```python
from build123d import *

# Parameters (mm, degrees)
SKETCH_8_W              = 3.5
SKETCH_8_H              = 303
SM_BASE_FLANGE_3_DEPTH  = 1.5
SM_EDGE_FLANGE_4_DEPTH  = 303
SM_EDGE_FLANGE_9_DEPTH  = 303
SM_EDGE_FLANGE_10_DEPTH = 303
FILLET_1_R              = 2


# Sheet-metal steps are written as plain solids
with BuildPart() as part:
    # Эскиз8 → Базовая кромка3 (new body)
    with BuildSketch(Plane.XY):
        with Locations((1.75, 151.5)):
            Rectangle(SKETCH_8_W, SKETCH_8_H)
    extrude(amount=-SM_BASE_FLANGE_3_DEPTH)

    # Ребро-кромка4 section (across the edge) → Ребро-кромка4 (add)
    with BuildSketch(Plane(origin=(32, 0, 0), x_dir=(-1, 0, 0), z_dir=(0, 1, 0))):
        with BuildLine():
            Line((-1.5, 28.5), (-1.5, 35))
            Line((-1.5, 35), (0, 35))
            Line((0, 35), (0, 28.5))
            ThreePointArc((0, 28.5), (8.347456736, 8.347456736), (28.5, 0))
            Line((28.5, 0), (28.5, -1.5))
            ThreePointArc((28.5, -1.5), (7.286796564, 7.286796564), (-1.5, 28.5))
        make_face()
    extrude(amount=SM_EDGE_FLANGE_4_DEPTH)

    # Ребро-кромка9 section (across the edge) → Ребро-кромка9 (add)
    with BuildSketch(Plane(origin=(-2, 303, 0), x_dir=(1, 0, 0), z_dir=(0, -1, 0))):
        with BuildLine():
            Line((-1.5, 2), (-1.5, 16.5))
            Line((-1.5, 16.5), (0, 16.5))
            Line((0, 16.5), (0, 2))
            ThreePointArc((0, 2), (0.585786438, 0.585786438), (2, 0))
            Line((2, 0), (2, -1.5))
            ThreePointArc((2, -1.5), (-0.474873734, -0.474873734), (-1.5, 2))
        make_face()
    extrude(amount=SM_EDGE_FLANGE_9_DEPTH)

    # Ребро-кромка10 section (across the edge) → Ребро-кромка10 (add)
    with BuildSketch(Plane(origin=(32, 0, 37), x_dir=(0, 0, -1), z_dir=(0, 1, 0))):
        with BuildLine():
            Line((-1.5, 2), (-1.5, 16.5))
            Line((-1.5, 16.5), (0, 16.5))
            Line((0, 16.5), (0, 2))
            ThreePointArc((0, 2), (0.585786438, 0.585786438), (2, 0))
            Line((2, 0), (2, -1.5))
            ThreePointArc((2, -1.5), (-0.474873734, -0.474873734), (-1.5, 2))
        make_face()
    extrude(amount=SM_EDGE_FLANGE_10_DEPTH)

    # Скругление1
    fillet_1_edges = [part.edges().sort_by_distance(p)[0] for p in [
        (-2.75, 303, 16.5),
        (-2.75, 0, 16.5),
        (15.5, 0, 37.75),
        (15.5, 303, 37.75),
    ]]
    fillet(fillet_1_edges, radius=FILLET_1_R)


solid = part.part
```
The listing builds one solid part. Answer for the finished solid, in the listing's coordinates (mm). A direction names the side the tool comes from. Give positions to 0.01 mm unless a question says otherwise; leave off trailing zeros. Loops run counter-clockwise (first coordinate to the right, second up) from the corner with the lowest first, then second, coordinate; pieces in that order, holes last. Notation, with made-up numbers: M 40,34 L 97,34 A25 cw 97,61 Z; hole C -32.5,15.25 d11. An arc over 180 degrees is marked long. One line per item, written item: value.
Q1. Flat-ended cylindrical pins translate along their axes: P1, Ø16, axis at y = 176.5, z = 5.5, coming from the +X side; P2, Ø2, axis at y = 187.5, z = 31, coming from the -X side; P3, Ø1.5, axis at y = 63, z = 24, coming from the -X side. Find the tip coordinate at first contact, or state that the pin passes through.
Working result:
P1: stops at x = 29.48
P2: stops at x = 32
P3: stops at x = 31.51
Q2. A cutting plane is placed at B-B on x = 22. Determine the outline of the cut face in (y, z), then the cut area to 3 significant figures.
Working result:
outline: M 0,4.88 L 303,4.88 L 303,6.82 L 0,6.82 Z; M 0,37 L 303,37 L 303,38.5 L 0,38.5 Z
area: 1,040 mm^2
Q3. A cutting plane is placed at D-D on z = 22. Determine the outline of the cut face in (x, y).
Working result:
outline: M 31.25,0 L 32.79,0 L 32.79,303 L 31.25,303 Z
Q4. A cutting plane is placed at C-C on y = 56. Determine the outline of the cut face in (x, z).
Working result:
outline: M -3.5,2 A3.5 ccw 0,-1.5 L 3.5,-1.5 A30 ccw 33.5,28.5 L 33.5,35 A3.5 ccw 30,38.5 L 15.5,38.5 L 15.5,37 L 30,37 A2 cw 32,35 L 32,28.5 A28.5 cw 3.5,0 L 0,0 A2 cw -2,2 L -2,16.5 L -3.5,16.5 Z
Q5. Find the intervals of material crossed by line 1 (X direction, y = 114, z = 28.5); line 2 (Z direction, x = 22.5, y = 221.5); line 3 (Z direction, x = 27.5, y = 132), in increasing order. Write a range as from..to.
Working result:
line 1: x = 32..33.5
line 2: z = 5.28..7.26, 37..38.5
line 3: z = 10.5..13.13, 37..38.5
Q6. A cutting plane is placed at A-A on z = 11. Determine the outline of the cut face in (x, y).
Working result:
outline: M -3.5,0 L -2,0 L -2,303 L -3.5,303 Z; M 25.99,0 L 27.87,0 L 27.87,303 L 25.99,303 Z
Q7. Determine the mould class of faces 1 (the face through (-2, 154, 9)), 2 (the face through (24.479, 149.379, 7.055)), 3 (the face through (25, 0, 8)) for opening direction X: +X half, -X half, draft (parallel to the pull), parting line (faces both ways), or undercut.
Working result:
face 1: undercut
face 2: +X half
face 3: draft
Q8. For faces 4 (the face through (23.9, 149.4, 8.6)), 5 (the face through (23, 149, 38.5)), 6 (the face through (32, 149, 32)), determine the directions among +Z, -Z, +X, -X, +Y, -Y from which every point of the face is accessible in a straight line to the end or side of a thin tool.
Working result:
face 4: +Y, -Y
face 5: +Z, +X, -X, +Y, -Y
face 6: -X, +Y, -Y
